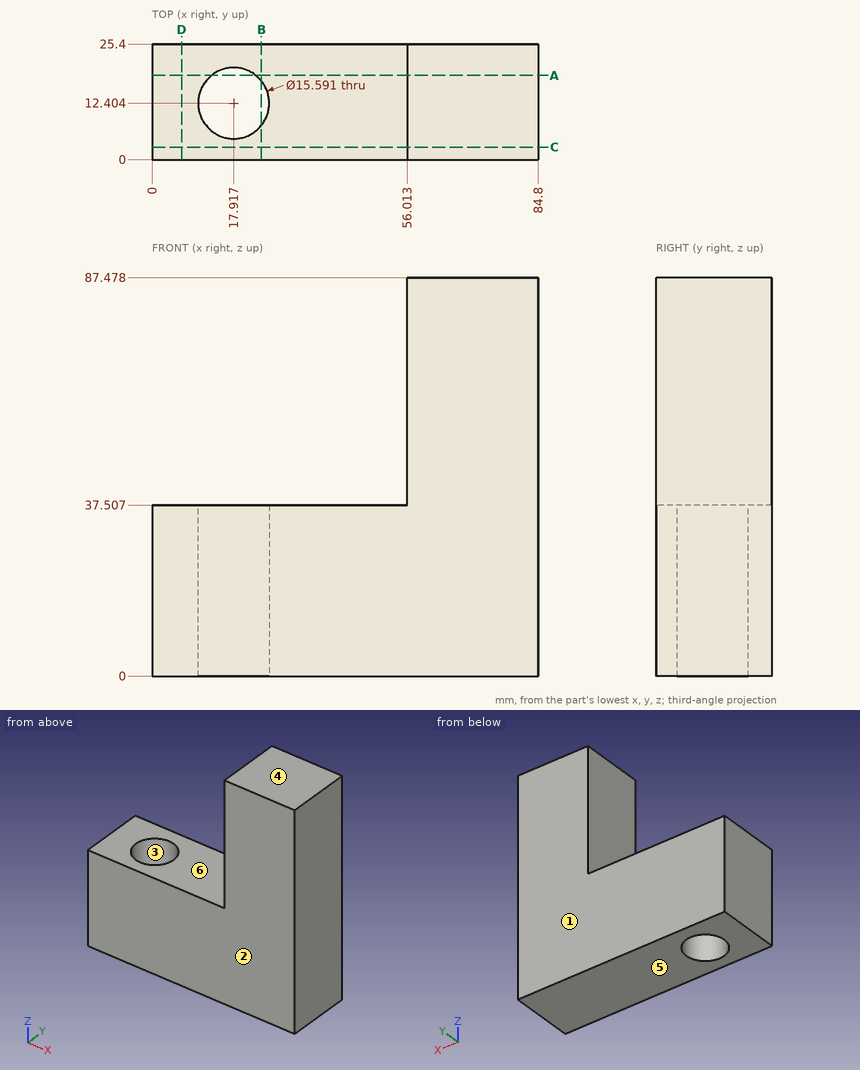
Geometry: see drawing. Coordinates: mm, zero at the bounding-box minimum. A direction names the side the tool comes from. Coordinates: 2 decimals unless noted, no trailing zeros. Order: outer loops, then holes, each group sorted by start corner. A loop starts at its lowest first (then second) coordinate and runs counter-clockwise, first axis right, second up. Notation, with made-up numbers: (37.25, 45.25) - (82.25, 45.25) arc R38 ccw to (82.25, 84.25) - close; hole circle Ø1 at (29, 12). An arc over 180 degrees is marked (long way). Write each question's results on one line, items separated by ' | '.
1) Section C-C, the plane y = 2.75. Return loops of the section in (x, z).
Results list:
outline: (0, 0) - (84.8, 0) - (84.8, 87.48) - (56.01, 87.48) - (56.01, 37.51) - (0, 37.51) - close
2) Pin query (flat end, axial travel): pin 1 (12.5 mm diameter, centred on x = 24.5, y = 18.5, fed in from +Z); pin 2 (12 mm diameter, centred on y = 14, z = 66, fed in from -X). Return the tip coordinate at first contact, or that it passes through.
Results list:
pin 1: z = 37.51 | pin 2: x = 56.01
3) Line query: line 1 (Y direction, x = 17.5, z = 22.5); line 2 (X direction, y = 6.25, z = 40.5); line 3 (Z direction, x = 24, y = 23.25). Output: solid intervals per line, ascending. Write a range as from..to.
Results list:
line 1: 0..4.62, 20.19..25.4 | line 2: 56.01..84.8 | line 3: 0..37.51
4) Section D-D, the plane x = 6.5. Return loops of the section in (y, z).
Results list:
outline: (0, 0) - (25.4, 0) - (25.4, 37.51) - (0, 37.51) - close
5) Set-up query: the marked faces 5 and 6. Return all of +Z, -Z, +X, -X, +Y, -Y with unobstructed straight access to the full face (end or side cutting, diameter ignored); none if empty.
Results list:
face 5: -Z, +X, -X, +Y, -Y | face 6: +Z, -X, +Y, -Y
6) Pull-direction query (Y, two-part tool) for the marked faces 1, 2, 3 and 4; classes: pulls with the +Y half, pulls with the -Y half, needs draft (parallel to the pull), parting line crosses it, or undercut.
Results list:
face 1: pulls with the +Y half | face 2: pulls with the -Y half | face 3: undercut | face 4: needs draft
7) Section A-A, the plane y = 18.5. Return loops of the section in (x, z).
Results list:
outline: (0, 0) - (13.06, 0) - (13.06, 37.51) - (0, 37.51) - close; (22.78, 0) - (84.8, 0) - (84.8, 87.48) - (56.01, 87.48) - (56.01, 37.51) - (22.78, 37.51) - close
8) Section B-B, the plane x = 24. Return loops of the section in (y, z).
Results list:
outline: (0, 0) - (7.53, 0) - (7.53, 37.51) - (0, 37.51) - close; (17.28, 0) - (25.4, 0) - (25.4, 37.51) - (17.28, 37.51) - close
